```python
from build123d import *

# Parameters (mm, degrees)
BOSS_EXTRUDE1_DEPTH     = 3
SKETCH4_W               = 40
SKETCH4_H               = 54
BOSS_EXTRUDE2_DEPTH     = 3
SKETCH11_W              = 3.9
SKETCH11_H              = 54
BOSS_EXTRUDE3_DEPTH     = 25
SKETCH16_R              = 2
SKETCH16_W              = 20
SKETCH16_H              = 40
CUT_EXTRUDE2_DEPTH      = 184.1
CUT_EXTRUDE2_DEPTH_BACK = 191.9
SKETCH13_R              = 2
SKETCH13_W              = 40
SKETCH13_H              = 20
CUT_EXTRUDE3_DEPTH      = 211.382685902
CUT_EXTRUDE3_DEPTH_BACK = 281.5
SKETCH12_R              = 2
SKETCH12_W              = 40
SKETCH12_H              = 20
CUT_EXTRUDE4_DEPTH      = 281.5
CUT_EXTRUDE4_DEPTH_BACK = 211.382685902
SKETCH17_W              = 20
SKETCH17_H              = 30
CUT_EXTRUDE5_DEPTH      = 80


with BuildPart() as part:
    # Sketch2 → Boss-Extrude1 (new body)
    with BuildSketch(Plane.XY):
        Polygon((-187, 161.946750508), (187, 161.946750508), (0, -161.946750508), align=None)
    extrude(amount=BOSS_EXTRUDE1_DEPTH)

    # Sketch4 → Boss-Extrude2 (add)
    with BuildSketch(Plane.XY.offset(3)):
        Polygon((116.882685902, -13.5), (96.882685902, -48.141016151), (50.117314098, -21.141016151), (70.117314098, 13.5), align=None)
        Polygon((-116.882685902, -13.5), (-136.882685902, 21.141016151), (-90.117314098, 48.141016151), (-70.117314098, 13.5), align=None)
        with Locations((20, 161.946750508)):
            Rectangle(SKETCH4_W, SKETCH4_H)
    extrude(amount=BOSS_EXTRUDE2_DEPTH)

    # Sketch11 → Boss-Extrude3 (add)
    with BuildSketch(Plane.XY.offset(6)):
        Polygon((116.882685902, -13.5), (114.932685902, -16.877499075), (68.167314098, 10.122500925), (70.117314098, 13.5), align=None)
        Polygon((-116.882685902, -13.5), (-118.832685902, -10.122500925), (-72.067314098, 16.877499075), (-70.117314098, 13.5), align=None)
        with Locations((1.95, 161.946750508)):
            Rectangle(SKETCH11_W, SKETCH11_H)
    extrude(amount=BOSS_EXTRUDE3_DEPTH)

    # Sketch16 → Cut-Extrude2 (cut, two sides)
    with BuildSketch(Plane(origin=(3.9, 0, 0), x_dir=(0, 0, -1), z_dir=(1, 0, 0))) as cut_extrude2_sk:
        with Locations((-13.5, 186.446750508)):
            Circle(SKETCH16_R)
        with Locations((-23.5, 186.446750508)):
            Circle(SKETCH16_R)
        with Locations((-23.5, 137.446750508)):
            Circle(SKETCH16_R)
        with Locations((-13.5, 137.446750508)):
            Circle(SKETCH16_R)
        with Locations((-18.5, 161.946750508)):
            Rectangle(SKETCH16_W, SKETCH16_H)
    extrude(amount=CUT_EXTRUDE2_DEPTH, mode=Mode.SUBTRACT)
    extrude(cut_extrude2_sk.sketch, amount=-CUT_EXTRUDE2_DEPTH_BACK, mode=Mode.SUBTRACT)

    # Sketch13 → Cut-Extrude3 (cut, two sides)
    with BuildSketch(Plane(origin=(23.375, 40.486687627, 0), x_dir=(0.866025404, -0.5, 0), z_dir=(0.5, 0.866025404, 0))) as cut_extrude3_sk:
        with Locations((105.473375254, -22)):
            Circle(SKETCH13_R)
        with Locations((105.473375254, -12)):
            Circle(SKETCH13_R)
        with Locations((56.473375254, -12)):
            Circle(SKETCH13_R)
        with Locations((56.473375254, -22)):
            Circle(SKETCH13_R)
        with Locations((80.973375254, -17)):
            Rectangle(SKETCH13_W, SKETCH13_H)
    extrude(amount=CUT_EXTRUDE3_DEPTH, mode=Mode.SUBTRACT)
    extrude(cut_extrude3_sk.sketch, amount=-CUT_EXTRUDE3_DEPTH_BACK, mode=Mode.SUBTRACT)

    # Sketch12 → Cut-Extrude4 (cut, two sides)
    with BuildSketch(Plane(origin=(-23.375, 40.486687627, 0), x_dir=(0.866025404, 0.5, 0), z_dir=(0.5, -0.866025404, 0))) as cut_extrude4_sk:
        with Locations((-56.473375254, 10.981481481)):
            Circle(SKETCH12_R)
        with Locations((-56.473375254, 20.981481481)):
            Circle(SKETCH12_R)
        with Locations((-105.473375254, 20.981481481)):
            Circle(SKETCH12_R)
        with Locations((-105.473375254, 10.981481481)):
            Circle(SKETCH12_R)
        with Locations((-80.973375254, 15.981481481)):
            Rectangle(SKETCH12_W, SKETCH12_H)
    extrude(amount=CUT_EXTRUDE4_DEPTH, mode=Mode.SUBTRACT)
    extrude(cut_extrude4_sk.sketch, amount=-CUT_EXTRUDE4_DEPTH_BACK, mode=Mode.SUBTRACT)

    # Sketch17 → Cut-Extrude5 (cut, symmetric)
    with BuildSketch(Plane.XY.offset(3)):
        Polygon((-93.5, 0), (-67.519237886, 15), (-57.519237886, -2.320508076), (-83.5, -17.320508076), align=None)
        Polygon((93.5, 0), (103.5, 17.320508076), (77.519237886, 32.320508076), (67.519237886, 15), align=None)
        with Locations((-10, 146.946750508)):
            Rectangle(SKETCH17_W, SKETCH17_H)
    extrude(amount=CUT_EXTRUDE5_DEPTH, both=True, mode=Mode.SUBTRACT)


solid = part.part
```
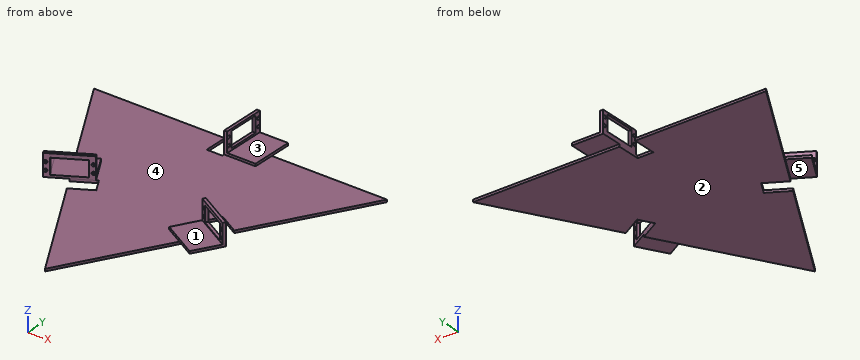
Here's how the part is built. I have some questions about the finished solid (model axes, mm). Face numbers are marked on the shaded views. A direction names the side the tool comes from. Give positions to 0.01 mm unless a question says otherwise; leave off trailing zeros. Order: outer loops, then holes, each group sorted by start corner. A loop starts at its lowest first (then second) coordinate and runs counter-clockwise, first axis right, second up. Notation, with made-up numbers: (12.25, -15.75) - (70.25, -15.75) arc R8 cw to (70.25, -10.75) - close; hole circle Ø7 at (-32.75, -23). An arc over 180 degrees is marked (long way). Answer as a JSON object with one key per item and string values. Group by question number.
Item 1: If we mould it in two halves opening along X, with no side actions, what happens to the marked faces 1 and 2? For each: pulls with the +X half, pulls with the -X half, needs draft (parallel to the pull), parting line crosses it, or undercut.
Item 2: For P1, Ø0.9, axis at y = 165, z = 4, coming from the +X side; P2, Ø1, axis at y = -8, z = 14, coming from the +X side; P3, Ø6, axis at x = -118.5, y = 85.5, coming from the +Z side; P4, Ø3.5, axis at y = 186.45, z = 23.5, coming from the -X side, each with a flat end and sliding along its axis, tell me the tip position at first contact or that it passes through.
Item 3: If we section it at A-A on y = 79.5: Please give me the cut outline in (x, z), and give its area (3 significant figures).
Item 4: Which directions (+Z, -Z, +X, -X, +Y, -Y) give clear straight access to the entire face, cutting with the end or side of a thin tool? Please do the marked faces 3, 4 and 5.
Item 5: Please list where these lines run through material, in increasing order: probe 1 along Y at (x, z) = (1.5, 23.5); probe 2 along Z at (x, y) = (-147.5, 153); probe 3 along Z at (x, y) = (75.5, -13).
Item 6: If we section it at B-B on x = -8: Please give me the cut outline in (y, z), and give its area (3 significant figures).
Result set:
{
 "1": {"face 1": "undercut", "face 2": "needs draft"},
 "2": {"P1": "x = 40", "P2": "x = -111.69", "P3": "z = 3", "P4": "through"},
 "3": {"outline": "(-139.4, 0) - (139.4, 0) - (139.4, 3) - (-139.4, 3) - close", "area": "836 mm²"},
 "4": {"face 3": "+Z, +X, +Y, -Y", "face 4": "+Z", "face 5": "-Z, -X, -Y"},
 "5": {"probe 1": "134.95 to 135.45, 139.45 to 141.95, 181.95 to 184.45, 188.45 to 188.95", "probe 2": "0 to 3", "probe 3": "0 to 6"},
 "6": {"outline": "(-148.09, 0) - (131.95, 0) - (131.95, 3) - (-148.09, 3) - close", "area": "840 mm²"}
}
